from build123d import *

# Parameters (mm, degrees)
EXTRUDE_1_DEPTH          = 3
SKETCH_2_OUTSIDE_W       = 13.724
SKETCH_2_OUTSIDE_H       = 8.024
CUT_EXTRUDE_1_DEPTH      = 12
SKETCH_3_R               = 1.05
CUT_EXTRUDE_2_DEPTH      = 12
FILLET_1_R               = 1
SKETCH_4_R               = 0.95
EXTRUDE_2_DEPTH          = 2
SKETCH_5_W               = 8
SKETCH_5_H               = 3
EXTRUDE_3_DEPTH          = 6
SKETCH_6_R               = 1.05
CUT_EXTRUDE_3_DEPTH      = 12
CUT_EXTRUDE_4_DEPTH      = 8
EXTRUDE_5_DEPTH          = 2
SKETCH_13_W              = 8
SKETCH_13_H              = 3
EXTRUDE_8_DEPTH          = 2
SKETCH_14_W              = 4
SKETCH_14_H              = 6
CUT_EXTRUDE_5_DEPTH      = 10
CUT_EXTRUDE_6_DEPTH      = 15.773286703
CUT_EXTRUDE_6_DEPTH_BACK = 15.773286703
SKETCH_11_R              = 1.05


with BuildPart() as part:
    # 草图1 → 凸台-拉伸1 (new body)
    with BuildSketch(Plane(origin=(0, 0, 0), x_dir=(1, 0, 0), z_dir=(0, 1, 0))):
        Polygon((-6, 0), (6, 0), (6, -8.7), (4, -8.7), (4, -3), (-4, -3), (-4, -8.7), (-6, -8.7), align=None)
    extrude(amount=EXTRUDE_1_DEPTH)

    # 草图2 outside → 切除-拉伸1 (cut)
    with BuildSketch(Plane.ZY.offset(6)):
        with Locations((4.35, 1.5)):
            Rectangle(SKETCH_2_OUTSIDE_W, SKETCH_2_OUTSIDE_H)
        with BuildLine():
            Line((6.2, 3), (0, 3))
            Line((0, 3), (0, 0))
            Line((0, 0), (6.2, 0))
            ThreePointArc((6.2, 0), (7.7, 1.5), (6.2, 3))
        make_face(mode=Mode.SUBTRACT)
    extrude(amount=-CUT_EXTRUDE_1_DEPTH, mode=Mode.SUBTRACT)

    # 草图3 → 切除-拉伸2 (cut)
    with BuildSketch(Plane.ZY.offset(6)):
        with Locations((5.2, 1.5)):
            Circle(SKETCH_3_R)
    extrude(amount=-CUT_EXTRUDE_2_DEPTH, mode=Mode.SUBTRACT)

    # 圆角1
    fillet_1_edges = [part.edges().sort_by_distance(p)[0] for p in [
        (-6, 1.5, 0),
        (6, 1.5, 0),
    ]]
    fillet(fillet_1_edges, radius=FILLET_1_R)

    # 草图4 → 凸台-拉伸2 (add)
    with BuildSketch(Plane(origin=(0, 0, 0), x_dir=(-1, 0, 0), z_dir=(0, 0, -1))):
        with Locations(Location((0, 1.5, 0), (0, 0, 180))):
            Circle(SKETCH_4_R)
    extrude(amount=EXTRUDE_2_DEPTH)

    # 草图5 → 凸台-拉伸3 (add)
    with BuildSketch(Plane(origin=(0, 0, -2), x_dir=(-1, 0, 0), z_dir=(0, 0, -1))):
        with Locations((0, 1.5)):
            Rectangle(SKETCH_5_W, SKETCH_5_H)
    extrude(amount=EXTRUDE_3_DEPTH)

    # 草图6 → 切除-拉伸3 (cut)
    with BuildSketch(Plane(origin=(4, 0, 0), x_dir=(0, 0, -1), z_dir=(1, 0, 0))):
        with Locations(Location((6, 1.5, 0), (0, 0, 90))):
            Circle(SKETCH_6_R)
    extrude(amount=-CUT_EXTRUDE_3_DEPTH, mode=Mode.SUBTRACT)

    # 草图8 → 切除-拉伸4 (cut)
    with BuildSketch(Plane(origin=(0, 3, 0), x_dir=(1, 0, 0), z_dir=(0, 1, 0))):
        Polygon((-1.5, 8), (1.5, 8), (2, 8), (2, 6), (1.5, 6), (-1.5, 6), (-2, 6), (-2, 8), align=None)
    extrude(amount=-CUT_EXTRUDE_4_DEPTH, mode=Mode.SUBTRACT)

    # 草图10 → 凸台-拉伸5 (add)
    with BuildSketch(Plane.ZY.offset(4)):
        with BuildLine():
            Line((-8, 3), (-8, 7.5))
            ThreePointArc((-8, 7.5), (-6, 9.5), (-4, 7.5))
            Line((-4, 7.5), (-4, 3))
            Line((-4, 3), (-8, 3))
        make_face()
    extrude_5 = extrude(amount=-EXTRUDE_5_DEPTH)

    # 镜向2: 凸台-拉伸5 across plane
    add(extrude_5.mirror(Plane(origin=(0, 0, 0), x_dir=(0, 0, 1), z_dir=(1, 0, 0))))

    # 草图13 → 凸台-拉伸8 (add)
    with BuildSketch(Plane.XY.offset(-2)):
        with Locations((0, 1.5)):
            Rectangle(SKETCH_13_W, SKETCH_13_H)
    extrude(amount=EXTRUDE_8_DEPTH)

    # 草图14 → 切除-拉伸5 (cut)
    with BuildSketch(Plane(origin=(0, 3, 0), x_dir=(1, 0, 0), z_dir=(0, 1, 0))):
        with Locations((0, 3)):
            Rectangle(SKETCH_14_W, SKETCH_14_H)
    extrude(amount=-CUT_EXTRUDE_5_DEPTH, mode=Mode.SUBTRACT)

    # 草图11 → 切除-拉伸6 (cut, two sides: drawn at the far end of the back side and taken through both)
    with BuildSketch(Plane.ZY.offset(2).offset(-CUT_EXTRUDE_6_DEPTH_BACK)):
        with Locations(Location((-6, 7.5, 0), (0, 0, 270))):
            Circle(SKETCH_11_R)
    extrude(amount=CUT_EXTRUDE_6_DEPTH + CUT_EXTRUDE_6_DEPTH_BACK, mode=Mode.SUBTRACT)


solid = part.part
Geometry check sheet. Reference: the model listing, model coordinates, mm. A direction names the side the tool comes from. Round coordinates to 2 decimals unless told otherwise and drop trailing zeros. Write each loop counter-clockwise with the first axis right and the second up, starting at its lowest first coordinate (ties: lowest second). Pieces come first, ordered by that corner, then holes. Notation, with made-up numbers: (17, 81) -> (55, 81) arc R24 cw to (55, 101) -> close; hole circle Ø9 at (-13, -2.75). An arc over 180 degrees is marked (long way). One line per item, written item: value. Start each with the question number.
(1) Draft check along X on faces 6 (the flat face through (-2, 4, -5)), 7 (the cylindrical face through (-5.699, 1.521, 0.285)), 8 (the flat face through (0, 3, 1)). Enter one of: +X half, -X half, draft (parallel to the pull), parting line (faces both ways), or undercut.
(2) Access from +Z, -Z, +X, -X, +Y, -Y to the whole of each face (thin tool, end or side, straight path). Record for faces 1 (the flat face through (-4.5, 1.5, 0)), 2 (the flat face through (-4, 2, 4)), 3 (the flat face through (-3, 5, -4)), 4 (the flat face through (0, 0, 1)), 5 (the flat face through (4.5, 1.5, 0)).
(3) Scan lines: line 1 (X direction, y = 2, z = -2); line 2 (Z direction, x = -3.35, y = 1.5); line 3 (Y direction, x = 5.5, z = 5.2). Record each from-to range of solid material in increasing order. Write a range as [from, to].
(4) Cross-section at C-C, the plane x = -3.5. Record the cut outline in (y, z), and give its area (3 significant figures).
(5) Cross-section at D-D, the plane z = -2. Record the cut outline in (x, y), and give its area (3 significant figures).
(6) Cross-section at B-B, the plane z = -6. Record the cut outline in (x, y).
(7) Go/stop test with flat-tipped pins: pin 1 Ø0.9 at (x, y) = (-1, 1.5) entering from -Z; pin 2 Ø2.5 at (y, z) = (5, -4.5) entering from -X; pin 3 Ø1 at (x, y) = (3, 5) entering from +Z. Record where each tip stops, or that it passes through.
(8) Cross-section at A-A, the plane y = 4.25. Record the cut outline in (x, z).
Answer:
1. face 6: undercut
1. face 7: -X half
1. face 8: draft
2. face 1: -Z, -X, +Y, -Y
2. face 2: +Z, +Y, -Y
2. face 3: +Z, +X, -X, +Y
2. face 4: +Z, -Z, +X, -X, -Y
2. face 5: -Z, +X, +Y, -Y
3. line 1: [-4, -2], [2, 4]
3. line 2: [-8, -7.05], [-4.95, 3]
3. line 3: [0, 0.45], [2.55, 3]
4. outline: (0, -8) -> (7.5, -8) arc R2 ccw to (7.5, -4) -> (3, -4) -> (3, 3) -> (0, 3) -> close; hole circle Ø2.1 at (1.5, -6); hole circle Ø2.1 at (7.5, -6)
4. area: 50.4 mm²
5. outline: (-4, 0) -> (-2, 0) -> (-2, 3) -> (-4, 3) -> close; (2, 0) -> (4, 0) -> (4, 3) -> (2, 3) -> close
5. area: 12.0 mm²
6. outline: (-4, 0) -> (-2, 0) -> (-2, 0.45) -> (-4, 0.45) -> close; (-4, 2.55) -> (-2, 2.55) -> (-2, 6.45) -> (-4, 6.45) -> close; (-4, 8.55) -> (-2, 8.55) -> (-2, 9.5) -> (-4, 9.5) -> close; (2, 0) -> (4, 0) -> (4, 0.45) -> (2, 0.45) -> close; (2, 2.55) -> (4, 2.55) -> (4, 6.45) -> (2, 6.45) -> close; (2, 8.55) -> (4, 8.55) -> (4, 9.5) -> (2, 9.5) -> close
7. pin 1: z = 0
7. pin 2: x = -4
7. pin 3: z = -4
8. outline: (-4, -8) -> (-2, -8) -> (-2, -4) -> (-4, -4) -> close; (2, -8) -> (4, -8) -> (4, -4) -> (2, -4) -> close
